from build123d import *

# Parameters (mm, degrees)
SKETCH1_W                   = 155
SKETCH1_H                   = 80
BOSS_EXTRUDE1_DEPTH         = 12.7
TAP_DRILL_FOR_M5X0_8_TAP1_D = 4.2


with BuildPart() as part:
    # Sketch1 → Boss-Extrude1 (new body)
    with BuildSketch(Plane(origin=(0, 0, 0), x_dir=(1, 0, 0), z_dir=(0, 1, 0))):
        Rectangle(SKETCH1_W, SKETCH1_H)
    extrude(amount=BOSS_EXTRUDE1_DEPTH)

    # Tap Drill for M5x0.8 Tap1 (through all)
    with Locations(Plane.XY.offset(40)):
        with Locations((-62.5, 6.35), (0, 6.35), (62.5, 6.35)):
            Hole(TAP_DRILL_FOR_M5X0_8_TAP1_D / 2)


solid = part.part
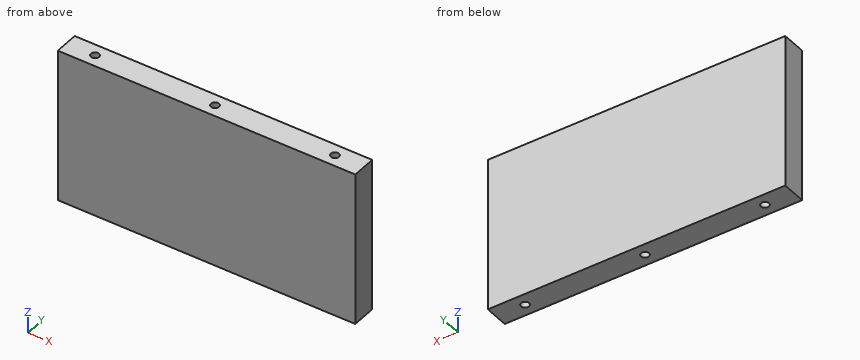
Here's how the part is built. I have some questions about the finished solid (model axes, mm). Round coordinates to 2 decimals unless told otherwise and drop trailing zeros. Order: outer loops, then holes, each group sorted by start corner. A loop starts at its lowest first (then second) coordinate and runs counter-clockwise, first axis right, second up. Notation, with made-up numbers: M 55,-29 L 89,-29 A32 ccw 89,2 Z; hole C 47,-38 d8. An arc over 180 degrees is marked long. Return JSON: item names as keys, results as strings. Group by question number.
1. If we section it at A-A on y = 6.35: List the corners of the cut face in (x, z) for me.
2. If we section it at B-B on z = -10: List the corners of the cut face in (x, y) for me, then the cut area to 3 significant figures.
3. Please list where these lines run through material, in increasing order: probe 1 along Y at (x, z) = (-62.5, -1); probe 2 along X at (y, z) = (8, 17).
4. If we section it at C-C on x = -62.5: List the corners of the cut face in (y, z) for me, then the cut area to 3 significant figures.
Reply:
{
 "1": {"outline": "M -77.5,-40 L -64.6,-40 L -64.6,40 L -77.5,40 Z; M -60.4,-40 L -2.1,-40 L -2.1,40 L -60.4,40 Z; M 2.1,-40 L 60.4,-40 L 60.4,40 L 2.1,40 Z; M 64.6,-40 L 77.5,-40 L 77.5,40 L 64.6,40 Z"},
 "2": {"outline": "M -77.5,0 L 77.5,0 L 77.5,12.7 L -77.5,12.7 Z; hole C -62.5,6.35 d4.2; hole C 0,6.35 d4.2; hole C 62.5,6.35 d4.2", "area": "1,930 mm^2"},
 "3": {"probe 1": "0 to 4.25, 8.45 to 12.7", "probe 2": "-77.5 to -63.8, -61.2 to -1.3, 1.3 to 61.2, 63.8 to 77.5"},
 "4": {"outline": "M 0,-40 L 4.25,-40 L 4.25,40 L 0,40 Z; M 8.45,-40 L 12.7,-40 L 12.7,40 L 8.45,40 Z", "area": "680 mm^2"}
}
